Here's the drawing with two shaded views (mm, measured from the low corner). I have some questions. A direction names the side the tool comes from. Give positions to 0.01 mm unless a question says otherwise; leave off trailing zeros. Loops run counter-clockwise (first coordinate to the right, second up) from the corner with the lowest first, then second, coordinate; pieces in that order, holes last. Notation, with made-up numbers: M 14,-2 L 44,-2 A13 cw 44,3 Z; hole C 63,29.25 d3. An arc over 180 degrees is marked long. Use CSV: the item, a comma, the result in double quotes.
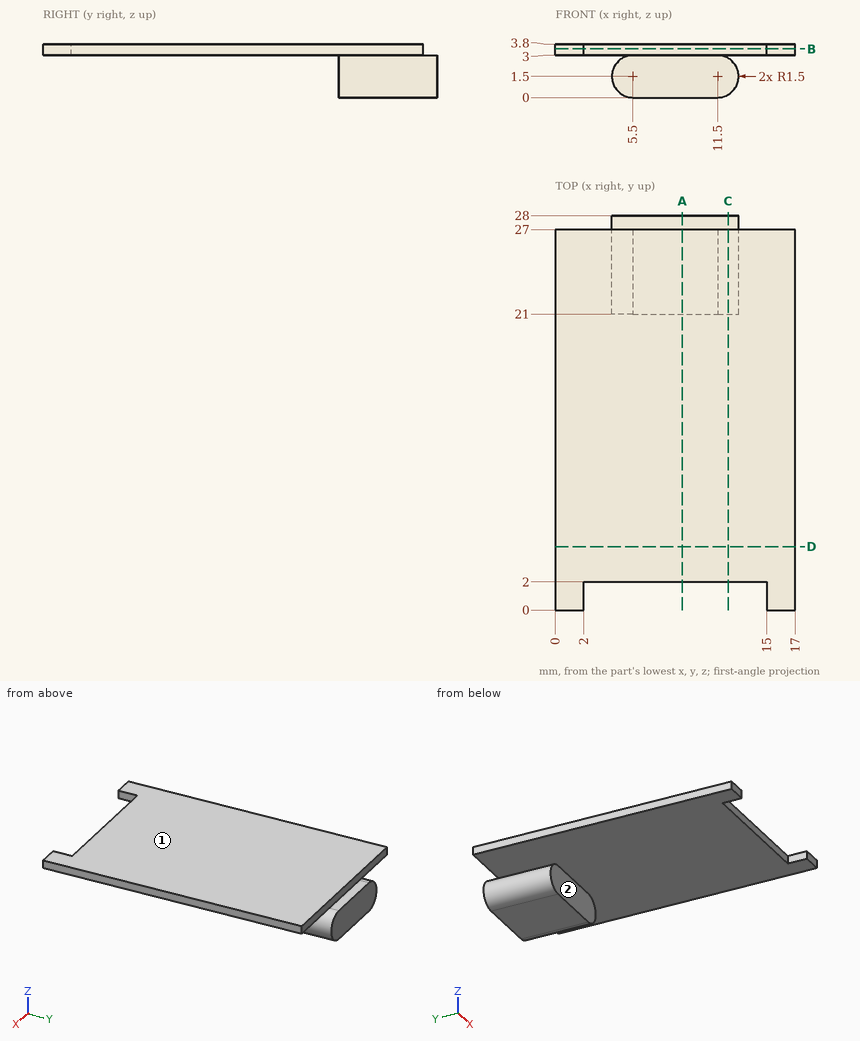
1. I want a section at C-C, the plane x = 12.25. List the corners of the cut face in (y, z) for me.
Outcome:
outline,"M 2,3 L 27,3 L 27,3.8 L 2,3.8 Z; M 21,0.2 L 28,0.2 L 28,2.8 L 21,2.8 Z"
2. Which directions (+Z, -Z, +X, -X, +Y, -Y) give clear straight access to the entire face, cutting with the end or side of a thin tool? Please do the marked faces 1 and 2.
Outcome:
face 1,"+Z, +X, -X, +Y, -Y"
face 2,"-Z, +X, -X, -Y"
3. I want a section at D-D, the plane y = 4.5. List the corners of the cut face in (x, z) for me.
Outcome:
outline,"M 0,3 L 17,3 L 17,3.8 L 0,3.8 Z"
4. I want a section at B-B, the plane z = 3.45. List the corners of the cut face in (x, y) for me, then the cut area to 3 significant figures.
Outcome:
outline,"M 0,0 L 2,0 L 2,2 L 15,2 L 15,0 L 17,0 L 17,27 L 0,27 Z"
area,"433 mm2"
5. Please list where these lines run through material, in increasing order: line 1 (Z direction, x = 5.5, y = 9.75); line 2 (Y direction, x = 6.5, z = 0.9); line 3 (Y direction, x = 16, z = 3.3).
Outcome:
line 1,"3 to 3.8"
line 2,"21 to 28"
line 3,"0 to 27"
6. I want a section at A-A, the plane x = 9. List the corners of the cut face in (y, z) for me.
Outcome:
outline,"M 2,3 L 21,3 L 21,0 L 28,0 L 28,3 L 27,3 L 27,3.8 L 2,3.8 Z"
7. I'm going to push flat-ended pins straight in: pin 1 Ø0.9 at (x, z) = (9, 1) entering from -Y; pin 2 Ø0.9 at (x, z) = (7.5, 3.5) entering from -Y; pin 3 Ø5 at (x, y) = (5, 17.5) entering from -Z. Where does each tip first touch, or does it pass through?
Outcome:
pin 1,"y = 21"
pin 2,"y = 2"
pin 3,"z = 3"
